from build123d import *

# Parameters (mm, degrees)
SKETCH_1_R          = 1.6
SKETCH_1_R_2        = 7.5
EXTRUDE_1_DEPTH     = 6.5
SKETCH_3_R          = 2.5
CUT_EXTRUDE_1_DEPTH = 68.222006253


with BuildPart() as part:
    # 草图1 → 凸台-拉伸1 (new body)
    with BuildSketch(Plane.XY):
        with BuildLine():
            Line((-36.800051208, 35), (38.850303739, 35))
            ThreePointArc((38.850303739, 35), (51.648918374, 29.698640239), (56.950278135, 16.900025604))
            Line((56.950278135, 16.900025604), (56.950278135, -16.900025604))
            ThreePointArc((56.950278135, -16.900025604), (50.945911029, -30.48186799), (36.800051208, -35))
            Line((36.800051208, -35), (-36.800051208, -35))
            ThreePointArc((-36.800051208, -35), (-49.598665842, -29.698640239), (-54.900025604, -16.900025604))
            Line((-54.900025604, -16.900025604), (-54.900025604, 16.900025604))
            ThreePointArc((-54.900025604, 16.900025604), (-49.598665842, 29.698640239), (-36.800051208, 35))
        make_face()
        with Locations(Location((-50.400025604, 16.900025604, 0), (0, 0, 180))):
            Circle(SKETCH_1_R, mode=Mode.SUBTRACT)
        with Locations(Location((-40.000025604, 10.900025604, 0), (0, 0, 180))):
            Circle(SKETCH_1_R_2, mode=Mode.SUBTRACT)
        with Locations(Location((52.450278135, 16.900025604, 0), (0, 0, 180))):
            Circle(SKETCH_1_R, mode=Mode.SUBTRACT)
        with Locations(Location((42.050278135, 10.900025604, 0), (0, 0, 180))):
            Circle(SKETCH_1_R_2, mode=Mode.SUBTRACT)
        with Locations(Location((52.450278135, -16.900025604, 0), (0, 0, 180))):
            Circle(SKETCH_1_R, mode=Mode.SUBTRACT)
        with Locations(Location((-50.400025604, -16.900025604, 0), (0, 0, 180))):
            Circle(SKETCH_1_R, mode=Mode.SUBTRACT)
        with BuildLine():
            Line((-15.5, 22.5), (15.5, 22.5))
            ThreePointArc((15.5, 22.5), (20.449747468, 20.449747468), (22.5, 15.5))
            Line((22.5, 15.5), (22.5, -15.5))
            ThreePointArc((22.5, -15.5), (20.449747468, -20.449747468), (15.5, -22.5))
            Line((15.5, -22.5), (-15.5, -22.5))
            ThreePointArc((-15.5, -22.5), (-20.449747468, -20.449747468), (-22.5, -15.5))
            Line((-22.5, -15.5), (-22.5, 15.5))
            ThreePointArc((-22.5, 15.5), (-20.449747468, 20.449747468), (-15.5, 22.5))
        make_face(mode=Mode.SUBTRACT)
    extrude(amount=EXTRUDE_1_DEPTH)

    # 草图3 → 切除-拉伸1 (cut, through all)
    with BuildSketch(Plane.XY.offset(6.5)):
        with Locations((-12, 28.75)):
            Circle(SKETCH_3_R)
        with Locations((12, 28.75)):
            Circle(SKETCH_3_R)
        with Locations((-6, -28.75)):
            Circle(SKETCH_3_R)
        with Locations((6, -28.75)):
            Circle(SKETCH_3_R)
    extrude(amount=-CUT_EXTRUDE_1_DEPTH, mode=Mode.SUBTRACT)


solid = part.part
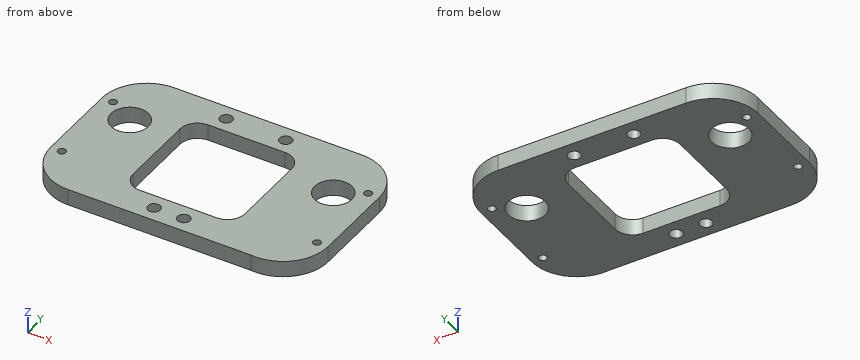
Could you check a few things on this model? Use its own coordinates, in mm. Coordinates: 2 decimals unless noted, no trailing zeros. Write each loop counter-clockwise with the first axis right and the second up, starting at its lowest first coordinate (ties: lowest second). Pieces come first, ordered by that corner, then holes. Notation, with made-up numbers: (34.5, -3.5) - (75.5, -3.5) arc R28 ccw to (75.5, 17.5) - close; hole circle Ø6 at (27.25, 50.5). An arc over 180 degrees is marked (long way). Put each result on its own line as item: value. Start each with the question number.
Q1. I want a section at B-B on y = -10.5. Write out the boundary of the cut face in (x, z).
Q2. Please list where these lines run through material, in increasing order: L1, parallel to Y at x = 6, z = 3; L2, parallel to Y at x = 12, z = 1.5; L3, parallel to X at y = -8.5, z = 2.75.
Q3. I want a section at A-A on x = 12. Write out the boundary of the cut face in (y, z), plus the area to 3 significant figures.
Q4. I want a section at D-D on y = 28.75. Write out the boundary of the cut face in (x, z), plus the area to 3 significant figures.
Q5. I want a section at C-C on x = 45. Write out the boundary of the cut face in (y, z), plus the area to 3 significant figures.
Q6. I'm going to push flat-ended pins straight in: P1, Ø6.5, axis at x = -12, y = 28.75, coming from the +Z side; P2, Ø3, axis at x = 42, z = 5.5, coming from the -Y side. Where does each tip first touch, or does it pass through?
Checks:
1. outline: (-54.9, 0) - (-22.5, 0) - (-22.5, 6.5) - (-54.9, 6.5) - close; (22.5, 0) - (56.95, 0) - (56.95, 6.5) - (22.5, 6.5) - close
2. L1: -35 to -31.25, -26.25 to -22.5, 22.5 to 35
2. L2: -35 to -22.5, 22.5 to 26.25, 31.25 to 35
2. L3: -54.9 to -22.5, 22.5 to 56.95
3. outline: (-35, 0) - (-22.5, 0) - (-22.5, 6.5) - (-35, 6.5) - close; (22.5, 0) - (26.25, 0) - (26.25, 6.5) - (22.5, 6.5) - close; (31.25, 0) - (35, 0) - (35, 6.5) - (31.25, 6.5) - close
3. area: 130 mm²
4. outline: (-50.48, 0) - (-14.5, 0) - (-14.5, 6.5) - (-50.48, 6.5) - close; (-9.5, 0) - (9.5, 0) - (9.5, 6.5) - (-9.5, 6.5) - close; (14.5, 0) - (52.53, 0) - (52.53, 6.5) - (14.5, 6.5) - close
4. area: 605 mm²
5. outline: (-34.04, 0) - (4, 0) - (4, 6.5) - (-34.04, 6.5) - close; (17.8, 0) - (33.92, 0) - (33.92, 6.5) - (17.8, 6.5) - close
5. area: 352 mm²
6. P1: z = 6.5
6. P2: y = -35.04
